Geometry: final body of the model. Coordinates: model frame, mm. Give positions to 0.01 mm unless a question says otherwise; leave off trailing zeros. Write each loop counter-clockwise with the first axis right and the second up, starting at its lowest first coordinate (ties: lowest second). Pieces come first, ordered by that corner, then holes. Notation, with made-up numbers: (63.5, 75.25) -> (78.5, 75.25) arc R22 cw to (78.5, 87.25) -> close; hole circle Ø11 at (-38, 21). An arc over 180 degrees is marked (long way). Answer in a Markdown table with one row per item. Add a question column.
Item 1: Material intervals for probe 1 along X at (y, z) = (137.7, 1); probe 2 along X at (y, z) = (-137.7, 2.7); probe 3 along Y at (x, z) = (237.7, 3.1), sorted ascending. Write a range as from..to.
Item 2: Section query D-D on x = -136.5. Output: boundary loops of the cut face in (y, z), plus the area to 3 significant figures.
Item 3: First-contact query: P1, Ø2.5, axis at x = -55, z = 2.5, coming from the +Y side; P2, Ø1, axis at x = 193, y = 66, coming from the -Z side. Flat tips, straight axial feed; report the tip coordinate or a pass-through.
Item 4: Section query B-B on x = -55. Output: boundary loops of the cut face in (y, z).
Item 5: Section query A-A on y = 54. Output: boundary loops of the cut face in (x, z), plus the area to 3 significant figures.
Item 6: Section query C-C on y = -67. State how many separate pieces and enclosed holes the cut face has, plus the area to 3 significant figures.
```python
from build123d import *

# Parameters (mm, degrees)
SKETCH_1_W          = 500.8
SKETCH_1_H          = 300.8
EXTRUDE_1_DEPTH     = 4.75
SKETCH_2_W          = 25.4
SKETCH_2_H          = 25.4
SKETCH_2_H_2        = 300.8
SKETCH_2_W_2        = 4.75
SKETCH_2_H_3        = 80
CUT_EXTRUDE_1_DEPTH = 10
SKETCH_3_R          = 2.15
SKETCH_3_R_2        = 2.150000004
CUT_EXTRUDE_2_DEPTH = 5
SKETCH_5_W          = 35
SKETCH_5_H          = 60
SKETCH_5_W_2        = 300
SKETCH_5_H_2        = 30
CUT_EXTRUDE_3_DEPTH = 10
FILLET_1_R          = 7


with BuildPart() as part:
    # 草圖1 → 填料-伸長1 (new body)
    with BuildSketch(Plane.XY):
        Rectangle(SKETCH_1_W, SKETCH_1_H)
    extrude(amount=EXTRUDE_1_DEPTH)

    # 草圖2 → 除料-伸長1 (cut)
    with BuildSketch(Plane(origin=(0, 0, 0), x_dir=(-1, 0, 0), z_dir=(0, 0, -1))):
        with Locations((-237.7, 137.7)):
            Rectangle(SKETCH_2_W, SKETCH_2_H)
        with Locations((-237.7, -137.7)):
            Rectangle(SKETCH_2_W, SKETCH_2_H)
        with Locations((237.7, 0)):
            Rectangle(SKETCH_2_W, SKETCH_2_H_2)
        with Locations((-222.625, 65.4)):
            Rectangle(SKETCH_2_W_2, SKETCH_2_H_3)
        with Locations((-222.625, -65.4)):
            Rectangle(SKETCH_2_W_2, SKETCH_2_H_3)
        with Locations((172.625, 65.4)):
            Rectangle(SKETCH_2_W_2, SKETCH_2_H_3)
        with Locations((172.625, -64.4)):
            Rectangle(SKETCH_2_W_2, SKETCH_2_H_3)
        with Locations((-127.375, 65.4)):
            Rectangle(SKETCH_2_W_2, SKETCH_2_H_3)
        with Locations((-72.625, 65.4)):
            Rectangle(SKETCH_2_W_2, SKETCH_2_H_3)
        with Locations((22.625, 65.4)):
            Rectangle(SKETCH_2_W_2, SKETCH_2_H_3)
        with Locations((77.375, 65.4)):
            Rectangle(SKETCH_2_W_2, SKETCH_2_H_3)
        with Locations((77.375, -65.4)):
            Rectangle(SKETCH_2_W_2, SKETCH_2_H_3)
        with Locations((22.625, -65.4)):
            Rectangle(SKETCH_2_W_2, SKETCH_2_H_3)
        with Locations((-127.375, -65.4)):
            Rectangle(SKETCH_2_W_2, SKETCH_2_H_3)
        with Locations((-72.625, -65.4)):
            Rectangle(SKETCH_2_W_2, SKETCH_2_H_3)
    extrude(amount=-CUT_EXTRUDE_1_DEPTH, mode=Mode.SUBTRACT)

    # 草圖3 → 除料-伸長2 (cut)
    with BuildSketch(Plane.XY.offset(4.75)):
        with Locations((-207.3, 137.7)):
            Circle(SKETCH_3_R)
        with Locations((-182.8, 137.7)):
            Circle(SKETCH_3_R)
        with Locations((182.8, 137.7)):
            Circle(SKETCH_3_R)
        with Locations((207.3, 137.7)):
            Circle(SKETCH_3_R)
        with Locations((237.7, 107.3)):
            Circle(SKETCH_3_R)
        with Locations((237.7, 82.8)):
            Circle(SKETCH_3_R)
        with Locations((237.7, -82.800000014)):
            Circle(SKETCH_3_R_2)
        with Locations((237.7, -107.300000014)):
            Circle(SKETCH_3_R_2)
        with Locations((207.3, -137.7)):
            Circle(SKETCH_3_R)
        with Locations((182.8, -137.7)):
            Circle(SKETCH_3_R)
        with Locations((-207.3, -137.7)):
            Circle(SKETCH_3_R)
        with Locations((-182.8, -137.7)):
            Circle(SKETCH_3_R)
    extrude(amount=-CUT_EXTRUDE_2_DEPTH, mode=Mode.SUBTRACT)

    # 草圖5 → 除料-伸長3 (cut)
    with BuildSketch(Plane.XY.offset(4.75)):
        with Locations((100, -65.4)):
            Rectangle(SKETCH_5_W, SKETCH_5_H)
        with Locations((-50, -65.4)):
            Rectangle(SKETCH_5_W, SKETCH_5_H)
        with Locations((-200, -65.4)):
            Rectangle(SKETCH_5_W, SKETCH_5_H)
        with Locations((0, 135.4)):
            Rectangle(SKETCH_5_W_2, SKETCH_5_H_2)
    extrude(amount=-CUT_EXTRUDE_3_DEPTH, mode=Mode.SUBTRACT)

    # 圓角1
    fillet_1_edges = [part.edges().sort_by_distance(p)[0] for p in [
        (-150, 120.4, 2.375),
        (150, 120.4, 2.375),
        (-182.5, -35.4, 2.375),
        (-182.5, -95.4, 2.375),
        (-217.5, -95.4, 2.375),
        (-217.5, -35.4, 2.375),
        (-32.5, -35.4, 2.375),
        (-32.5, -95.4, 2.375),
        (-67.5, -95.4, 2.375),
        (-67.5, -35.4, 2.375),
        (117.5, -35.4, 2.375),
        (117.5, -95.4, 2.375),
        (82.5, -95.4, 2.375),
        (82.5, -35.4, 2.375),
    ]]
    fillet(fillet_1_edges, radius=FILLET_1_R)


solid = part.part
```
Findings below:
| question | item | result |
|---|---|---|
| 1 | probe 1 | x = -225..-209.45, -205.15..-184.95, -180.65..-150, 150..180.65, 184.95..205.15, 209.45..225 |
| 1 | probe 2 | x = -225..-209.45, -205.15..-184.95, -180.65..180.65, 184.95..205.15, 209.45..225 |
| 1 | probe 3 | y = -125..-109.45, -105.15..-84.95, -80.65..80.65, 84.95..105.15, 109.45..125 |
| 2 | outline | (-150.4, 0) -> (120.4, 0) -> (120.4, 4.75) -> (-150.4, 4.75) -> close |
| 2 | area | 1,290 mm^2 |
| 3 | P1 | stops at y = 120.4 |
| 3 | P2 | stops at z = 0 |
| 4 | outline | (-150.4, 0) -> (-95.4, 0) -> (-95.4, 4.75) -> (-150.4, 4.75) -> close; (-35.4, 0) -> (120.4, 0) -> (120.4, 4.75) -> (-35.4, 4.75) -> close |
| 5 | outline | (-225, 0) -> (-175, 0) -> (-175, 4.75) -> (-225, 4.75) -> close; (-170.25, 0) -> (-79.75, 0) -> (-79.75, 4.75) -> (-170.25, 4.75) -> close; (-75, 0) -> (-25, 0) -> (-25, 4.75) -> (-75, 4.75) -> close; (-20.25, 0) -> (70.25, 0) -> (70.25, 4.75) -> (-20.25, 4.75) -> close; (75, 0) -> (125, 0) -> (125, 4.75) -> (75, 4.75) -> close; (129.75, 0) -> (220.25, 0) -> (220.25, 4.75) -> (129.75, 4.75) -> close; (225, 0) -> (250.4, 0) -> (250.4, 4.75) -> (225, 4.75) -> close |
| 5 | area | 2,120 mm^2 |
| 6 | separate pieces | 10 |
| 6 | enclosed holes | 0 |
| 6 | area | 1,620 mm^2 |
